from build123d import *

# Parameters (mm, degrees)
F0_W     = 144
F0_H     = 300
F1_DEPTH = 6
F3_DEPTH = 0.1
F4_R     = 22.5
F4_R_2   = 32.5
F5_DEPTH = 25
F6_W     = 15
F6_H     = 6
F7_DEPTH = 25
F8_W     = 6
F8_H     = 15
F9_DEPTH = 25


with BuildPart() as f1:
    # F0 (on Right) → F1 (new body)
    with BuildSketch(Plane.YZ):
        Rectangle(F0_W, F0_H)
    extrude(amount=F1_DEPTH)

    # F2 (on face) → F3 (cut)
    with BuildSketch(Plane.YZ.offset(6)):
        Polygon((-75, 132), (75, 132), (75, 138), (0, 138), (-75, 138), align=None)
    extrude(amount=-F3_DEPTH, mode=Mode.SUBTRACT)

    # F4 (on face) → F5 (intersect)
    with BuildSketch(Plane.YZ.offset(6)):
        with BuildLine():
            add(Edge.make_bspline(
                [(-72, 119.5738017559), (-64.2497774345, 80.5000488248), (-48.1346297131, -0.7465599275), (-63.8451208348, -92.1644998818), (-72, -139.617010951)],
                knots=[0, 0, 0, 0, 0.4809278016, 1, 1, 1, 1], degree=3))
            ThreePointArc((-72, -139.617010951), (-69.2733831197, -147.3778685956), (-61.4766031504, -150))
            add(Edge.make_bspline(
                [(0, -144.7299867868), (-36.2115949392, -144.0225094557), (-40.9844021002, -148.2433289289), (-61.4766031504, -150)],
                knots=[0, 0, 0, 0, 61.7020726895, 61.7020726895, 61.7020726895, 61.7020726895], degree=3))
            add(Edge.make_bspline(
                [(0, -144.7299867868), (36.2115949392, -144.0225094557), (40.9844021002, -148.2433289289), (61.4766031504, -150)],
                knots=[0, 0, 0, 0, 61.7020726895, 61.7020726895, 61.7020726895, 61.7020726895], degree=3))
            ThreePointArc((61.4766031504, -150), (69.2733831197, -147.3778685956), (72, -139.617010951))
            add(Edge.make_bspline(
                [(72, 119.5738017559), (64.2497774345, 80.5000488248), (48.1346297131, -0.7465599275), (63.8451208348, -92.1644998818), (72, -139.617010951)],
                knots=[0, 0, 0, 0, 0.4809278016, 1, 1, 1, 1], degree=3))
            Line((72, 119.5738017559), (83.392560482, 131.8830251694))
            Line((83.392560482, 131.8830251694), (71.9000700982, 144.2635640774))
            ThreePointArc((71.9000700982, 144.2635640774), (70.0901190751, 148.7192160834), (65.4091020209, 149.8223193611))
            add(Edge.make_bspline(
                [(65.4091020209, 149.8223193611), (43.2062713991, 146.9935488104), (25.1373257488, 140.970274806), (0, 141.4896994829)],
                knots=[0, 0, 0, 0, 65.9377219898, 65.9377219898, 65.9377219898, 65.9377219898], degree=3))
            add(Edge.make_bspline(
                [(-65.4091020209, 149.8223193611), (-43.2062713991, 146.9935488104), (-25.1373257488, 140.970274806), (0, 141.4896994829)],
                knots=[0, 0, 0, 0, 65.9377219898, 65.9377219898, 65.9377219898, 65.9377219898], degree=3))
            ThreePointArc((-65.4091020209, 149.8223193611), (-70.0901190751, 148.7192160834), (-71.9000700982, 144.2635640774))
            Line((-71.9000700982, 144.2635640774), (-83.392560482, 131.8830251694))
            Line((-83.392560482, 131.8830251694), (-72, 119.5738017559))
        make_face()
        with Locations((0, -85)):
            Circle(F4_R, mode=Mode.SUBTRACT)
        Circle(F4_R_2, mode=Mode.SUBTRACT)
        with Locations((0, 85)):
            Circle(F4_R, mode=Mode.SUBTRACT)
    extrude(amount=-F5_DEPTH, mode=Mode.INTERSECT)

    # F6 (on face) → F7 (cut)
    with BuildSketch(Plane.YZ.offset(5.9)):
        with Locations((-47.5, 135)):
            Rectangle(F6_W, F6_H)
        with Locations((47.5, 135)):
            Rectangle(F6_W, F6_H)
    extrude(amount=-F7_DEPTH, mode=Mode.SUBTRACT)

    # F8 (on face) → F9 (cut)
    with BuildSketch(Plane.YZ.offset(6)):
        with Locations((59, 109.5)):
            Rectangle(F8_W, F8_H)
        with Locations((59, -109.5)):
            Rectangle(F8_W, F8_H)
        with Locations((-59, 109.5)):
            Rectangle(F8_W, F8_H)
        with Locations((-59, -109.5)):
            Rectangle(F8_W, F8_H)
    extrude(amount=-F9_DEPTH, mode=Mode.SUBTRACT)


solid = f1.part
Verification items for the finished model (mm, model axes). A direction names the side the tool comes from. Give positions to 0.01 mm unless a question says otherwise; leave off trailing zeros.
1) Depth check by flat-ended pin: pin 1 Ø3 at (x, z) = (4, -109.5) entering from +Y; pin 2 Ø1.8 at (x, z) = (2, 106.5) entering from +Y; pin 3 Ø1.8 at (y, z) = (-65, 133.5) entering from +X. Enter the tip coordinate at first touch or a pass-through.
2) Set-up check for faces 4 (the flat face through (3, -59, -117)), 5 (the flat face through (3, -72, 132)): record each of +Z, -Z, +X, -X, +Y, -Y from which the full face is reachable in a straight line by a thin tool's end or side.
3) Thickness scan on line 1 along Z through (x, y) = (1.5, 0); line 2 along Y through (x, z) = (4.25, -104); line 3 along Z through (x, y) = (5.5, -8.5). Record the ranges inside material, lowest first.
4) Sectioned sample at A-A, the plane y = -9. Count the separate pieces of the cut face and the enclosed holes in it, then the cut area to 3 significant figures.
5) Draft check along Z on faces 1 (the cylindrical face through (3.04, -69.42, -147.23)), 2 (the flat face through (0, -33, 2)), 3 (the flat face through (3, 62, 109)). Enter one of: pulls with the +Z half, pulls with the -Z half, needs draft (parallel to the pull), parting line crosses it, or undercut.
Answers:
1. pin 1: stops at y = 67.15
1. pin 2: stops at y = 69.59
1. pin 3: stops at x = 5.9
2. face 4: +X, -X
2. face 5: +Z, -Z, +X, -X, -Y
3. line 1: z = -144.73 to -107.5, -62.5 to -32.5, 32.5 to 62.5, 107.5 to 141.49
3. line 2: y = -66.01 to -62, -56 to -12.05, 12.05 to 56, 62 to 66.01
3. line 3: z = -144.65 to -105.83, -64.17 to -31.37, 31.37 to 64.17, 105.83 to 141.56
4. separate pieces: 4
4. enclosed holes: 0
4. area: 847 mm2
5. face 1: pulls with the -Z half
5. face 2: needs draft
5. face 3: undercut
